```python
from build123d import *

# Parameters (mm, degrees)
F1_DEPTH = 6.35


with BuildPart() as f1:
    # F0 (on Front) → F1 (new body)
    with BuildSketch(Plane.XZ):
        with BuildLine():
            ThreePointArc((0, 1.6), (1.1313708499, 1.1313708499), (1.6, 0))
            ThreePointArc((1.6, 0), (1.1313708499, -1.1313708499), (0, -1.6))
            Line((0, -1.6), (0, -3.175))
            ThreePointArc((0, -3.175), (2.2450640303, -2.2450640303), (3.175, 0))
            ThreePointArc((3.175, 0), (2.2450640303, 2.2450640303), (0, 3.175))
            Line((0, 3.175), (0, 1.6))
        make_face()
        with BuildLine():
            ThreePointArc((-1.6, 0), (-1.1313708499, 1.1313708499), (0, 1.6))
            Line((0, 1.6), (0, 3.175))
            ThreePointArc((0, 3.175), (-2.2450640303, 2.2450640303), (-3.175, 0))
            Line((-3.175, 0), (-1.6, 0))
        make_face()
        with BuildLine():
            Line((0, -3.175), (0, -1.6))
            ThreePointArc((0, -1.6), (-1.1313708499, -1.1313708499), (-1.6, 0))
            Line((-1.6, 0), (-3.175, 0))
            ThreePointArc((-3.175, 0), (-2.2450640303, -2.2450640303), (0, -3.175))
        make_face()
        with BuildLine():
            ThreePointArc((-3.175, 0), (-2.2450640303, 2.2450640303), (0, 3.175))
            Line((0, 3.175), (-128.2390823674, 3.1749812291))
            ThreePointArc((-128.2390823674, 3.1749812291), (-126.0010793162, 2.2412007403), (-125.075, 0))
            Line((-125.075, 0), (-3.175, 0))
        make_face()
        with BuildLine():
            Line((-128.25, -3.175), (0, -3.175))
            ThreePointArc((0, -3.175), (-2.2450640303, -2.2450640303), (-3.175, 0))
            Line((-3.175, 0), (-125.075, 0))
            ThreePointArc((-125.075, 0), (-126.0049359697, -2.2450640303), (-128.25, -3.175))
        make_face()
        with BuildLine():
            Line((-128.2417899522, 1.6001789385), (-128.2390823674, 3.1749812291))
            ThreePointArc((-128.2390823674, 3.1749812291), (-131.4249953073, 0.0054588244), (-128.25, -3.175))
            Line((-128.25, -3.175), (-128.2472924152, -1.6001977093))
            ThreePointArc((-128.2472924152, -1.6001977093), (-129.8501976349, 0.0027512475), (-128.2417899522, 1.6001789385))
        make_face()
        with BuildLine():
            ThreePointArc((-125.075, 0), (-126.0010793162, 2.2412007403), (-128.2390823674, 3.1749812291))
            Line((-128.2390823674, 3.1749812291), (-128.2417899522, 1.6001789385))
            ThreePointArc((-128.2417899522, 1.6001789385), (-127.1155887521, 1.1286058483), (-126.6498, 0))
            Line((-126.6498, 0), (-125.075, 0))
        make_face()
        with BuildLine():
            Line((-128.2472924152, -1.6001977093), (-128.25, -3.175))
            ThreePointArc((-128.25, -3.175), (-126.0049359697, -2.2450640303), (-125.075, 0))
            Line((-125.075, 0), (-126.6498, 0))
            ThreePointArc((-126.6498, 0), (-127.1175308575, -1.1305545902), (-128.2472924152, -1.6001977093))
        make_face()
    extrude(amount=F1_DEPTH)


solid = f1.part
```
The listing builds one solid part. Answer for the finished solid, in the listing's coordinates (mm). Give positions to 0.01 mm unless a question says otherwise; leave off trailing zeros. Order: outer loops, then holes, each group sorted by start corner. A loop starts at its lowest first (then second) coordinate and runs counter-clockwise, first axis right, second up. Notation, with made-up numbers: M 47,23 L 72,23 A22 cw 72,56 Z; hole C 79,-21 d5. An arc over 180 degrees is marked long. Put each result on its own line as item: value. Start each with the question number.
Item 1: A flat-ended cylindrical pin translates along its axis: P1, Ø2, axis at y = -4.5, z = -1, coming from the -X side (3 decimals). Find the tip coordinate at first contact, or state that the pin passes through.
Item 2: The part is cut by section A-A, the plane y = -5.25. Determine the outline of the cut face in (x, z) (3 decimals).
Item 3: Find the intervals of material crossed by line 1 along X through (y, z) = (-5.25, 0.75); line 2 along X through (y, z) = (-5.75, -0.5); line 3 along X through (y, z) = (-6, 2.75), in increasing order.
Answer key:
1. P1: stops at x = -131.425
2. outline: M -128.25,-3.175 L 0,-3.175 A3.175 ccw 0,3.175 L -128.239,3.175 A3.175 ccw Z; hole C -128.25,0 d3.2; hole C 0,0 d3.2
3. line 1: x = -131.34 to -129.66, -126.84 to -1.41, 1.41 to 3.09
3. line 2: x = -131.39 to -129.77, -126.73 to -1.52, 1.52 to 3.14
3. line 3: x = -129.84 to 1.59
